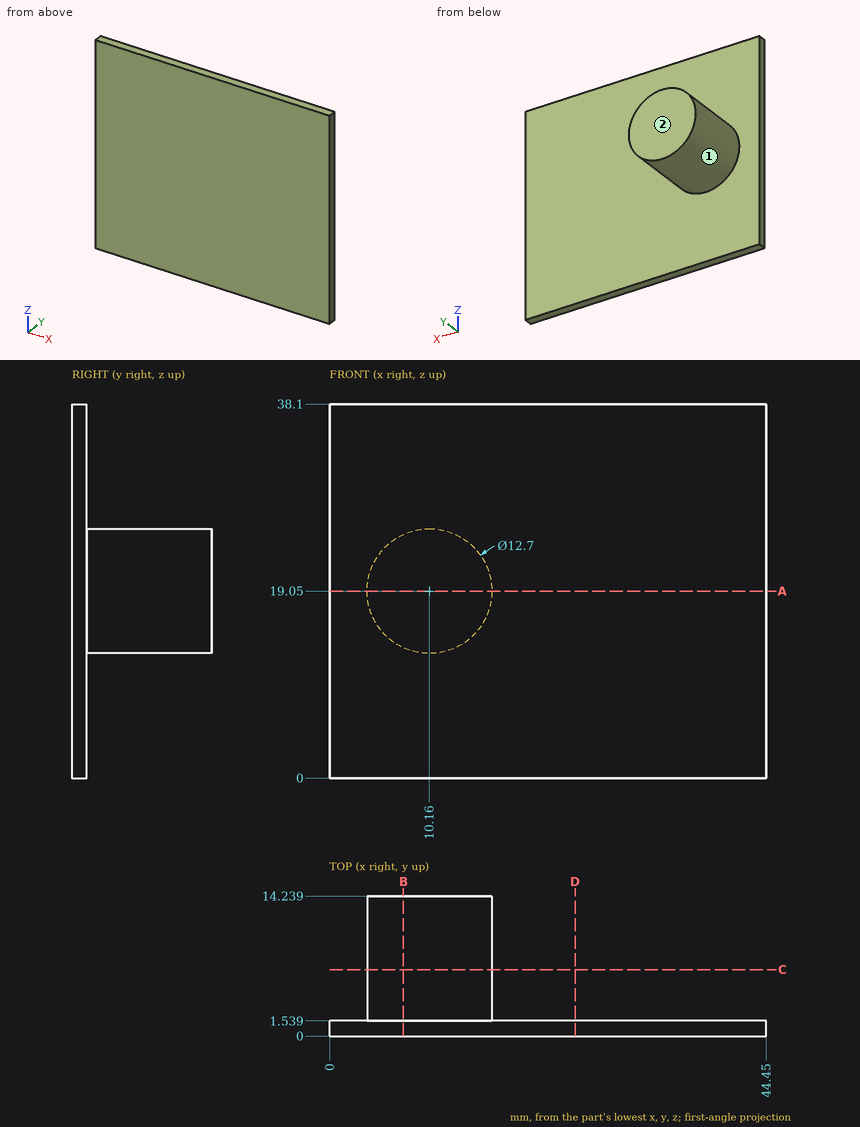
Geometry: see drawing. Coordinates: mm, zero at the bounding-box minimum. A direction names the side the tool comes from. Give positions to 0.01 mm unless a question says otherwise; leave off trailing zeros. Loops run counter-clockwise (first coordinate to the right, second up) from the corner with the lowest first, then second, coordinate; pieces in that order, holes last. Notation, with made-up numbers: (61.25, -7) - (77.25, -7) arc R27 ccw to (77.25, 12) - close; hole circle Ø1 at (65.5, -23). An arc over 180 degrees is marked (long way). Use CSV: the item, a comma, the result in double quotes. Start each with the question number.
1. Section B-B (x = 7.5). Output: boundary loops of the cut face in (y, z).
2. Pin query (flat end, axial travel): pin 1 (5 mm diameter, centred on x = 8, y = 9, fed in from -Z). Return the tip coordinate at first contact, or that it passes through.
3. Ray query, L1, parallel to Y at x = 32, z = 24; L2, parallel to X at y = 5.25, z = 15.5 (1 decimal); L3, parallel to Z at x = 11, y = 7.75. Return the intervals inside material, ascending.
4. Section D-D (x = 25). Output: boundary loops of the cut face in (y, z).
5. Reachability of the marked faces 1 and 2 from +Z, -Z, +X, -X, +Y, -Y: full face, straight path, thin tool, end or side. Return the list, or none.
6. Section C-C (y = 6.75). Output: boundary loops of the cut face in (x, z), then the cut area to 3 significant figures.
7. Section A-A (z = 19.05). Output: boundary loops of the cut face in (x, y).
Response:
1,outline,"(0, 0) - (1.54, 0) - (1.54, 13.28) - (14.24, 13.28) - (14.24, 24.82) - (1.54, 24.82) - (1.54, 38.1) - (0, 38.1) - close"
2,pin 1,"z = 12.7"
3,L1,"0 to 1.54"
3,L2,"4.9 to 15.4"
3,L3,"12.76 to 25.34"
4,outline,"(0, 0) - (1.54, 0) - (1.54, 38.1) - (0, 38.1) - close"
5,face 1,"+Y"
5,face 2,"+Z, -Z, +X, -X, +Y"
6,outline,"circle Ø12.7 at (10.16, 19.05)"
6,area,"127 mm²"
7,outline,"(0, 0) - (44.45, 0) - (44.45, 1.54) - (16.51, 1.54) - (16.51, 14.24) - (3.81, 14.24) - (3.81, 1.54) - (0, 1.54) - close"
